Build history of the part. All positions in model axes, mm. Give positions to 0.01 mm unless a question says otherwise; leave off trailing zeros. Order: outer loops, then holes, each group sorted by start corner. A loop starts at its lowest first (then second) coordinate and runs counter-clockwise, first axis right, second up. Notation, with made-up numbers: (-24.5, -28) - (13.5, -28) arc R27 cw to (13.5, -10) - close; hole circle Ø9 at (-27.75, 55). An arc over 180 degrees is marked (long way). Use a Markdown table: item, result. Add a question column.
(1) Slice it at B-B (z = 2.5). Count the separate pieces of the cut face and the enclosed holes in it, then the cut area to 3 significant figures.
(2) Slice it at D-D (x = 23.5). Write the cut outline in (y, z), then the cut area to 3 significant figures.
(3) Wall check: line 1 (X direction, y = 14.25, z = 6.25); line 2 (Y direction, x = 6.5, z = 5.75); line 3 (Y direction, x = 42.5, z = 7). Give the ranges that are in metal, low to high.
(4) Slice it at C-C (y = 23.25). Write the cut outline in (x, z).
(5) Mould opens along Y. For faces 1 (the face through (37.37, 11.62, 3.76)), 2 (the face through (22, 18, 0)), 3 (the face through (22, 28.419, 4)) say: +Y half, -Y half, draft (parallel to the pull), parting line (faces both ways), or undercut.
(6) Slice it at A-A (x = 13.5). Write the cut outline in (y, z), then the cut area to 3 significant figures.
from build123d import *

# Parameters (mm, degrees)
SKETCH1_W           = 45.596558684
SKETCH1_H           = 28.418694735
SKETCH1_R           = 3.675
SKETCH1_R_2         = 3.67
SKETCH1_R_3         = 3.665
SKETCH1_R_4         = 3.66
SKETCH1_R_5         = 3.655
SKETCH1_R_6         = 3.645
SKETCH1_R_7         = 3.64
SKETCH1_R_8         = 3.635
SKETCH1_R_9         = 3.63
SKETCH1_R_10        = 3.62
SKETCH1_R_11        = 3.615
SKETCH1_R_12        = 3.61
SKETCH1_R_13        = 3.605
SKETCH1_R_14        = 3.65
SKETCH1_R_15        = 3.625
BOSS_EXTRUDE1_DEPTH = 7.62
CHAMFER1_SIZE       = 2.54


with BuildPart() as part:
    # Sketch1 → Boss-Extrude1 (new body)
    with BuildSketch(Plane.XY):
        with Locations((22.798279342, 14.209347368)):
            Rectangle(SKETCH1_W, SKETCH1_H)
        with Locations((4.694723918, 4.934387692)):
            Circle(SKETCH1_R, mode=Mode.SUBTRACT)
        with Locations((13.584723918, 4.934387692)):
            Circle(SKETCH1_R_2, mode=Mode.SUBTRACT)
        with Locations((22.474723918, 4.934387692)):
            Circle(SKETCH1_R_3, mode=Mode.SUBTRACT)
        with Locations((31.364723918, 4.934387692)):
            Circle(SKETCH1_R_4, mode=Mode.SUBTRACT)
        with Locations((40.254723918, 4.934387692)):
            Circle(SKETCH1_R_5, mode=Mode.SUBTRACT)
        with Locations((13.584723918, 13.824387692)):
            Circle(SKETCH1_R_6, mode=Mode.SUBTRACT)
        with Locations((22.474723918, 13.824387692)):
            Circle(SKETCH1_R_7, mode=Mode.SUBTRACT)
        with Locations((31.364723918, 13.824387692)):
            Circle(SKETCH1_R_8, mode=Mode.SUBTRACT)
        with Locations((40.254723918, 13.824387692)):
            Circle(SKETCH1_R_9, mode=Mode.SUBTRACT)
        with Locations((13.584723918, 22.714387692)):
            Circle(SKETCH1_R_10, mode=Mode.SUBTRACT)
        with Locations((22.474723918, 22.714387692)):
            Circle(SKETCH1_R_11, mode=Mode.SUBTRACT)
        with Locations((31.364723918, 22.714387692)):
            Circle(SKETCH1_R_12, mode=Mode.SUBTRACT)
        with Locations((40.254723918, 22.714387692)):
            Circle(SKETCH1_R_13, mode=Mode.SUBTRACT)
        with Locations((4.694723918, 13.824387692)):
            Circle(SKETCH1_R_14, mode=Mode.SUBTRACT)
        with Locations((4.694723918, 22.714387692)):
            Circle(SKETCH1_R_15, mode=Mode.SUBTRACT)
    extrude(amount=BOSS_EXTRUDE1_DEPTH)

    # Chamfer1
    chamfer1_edges = [part.edges().sort_by_distance(p)[0] for p in [
        (0, 0, 3.81),
    ]]
    chamfer(chamfer1_edges, length=CHAMFER1_SIZE)


solid = part.part
Solution:
| question | item | result |
|---|---|---|
| 1 | separate pieces | 1 |
| 1 | enclosed holes | 15 |
| 1 | area | 668 mm2 |
| 2 | outline | (0, 0) - (1.42, 0) - (1.42, 7.62) - (0, 7.62) - close; (8.45, 0) - (10.33, 0) - (10.33, 7.62) - (8.45, 7.62) - close; (17.32, 0) - (19.25, 0) - (19.25, 7.62) - (17.32, 7.62) - close; (26.18, 0) - (28.42, 0) - (28.42, 7.62) - (26.18, 7.62) - close |
| 2 | area | 56.9 mm2 |
| 3 | line 1 | 0 to 1.07, 8.32 to 9.96, 17.2 to 18.86, 26.09 to 27.75, 34.97 to 36.65, 43.86 to 45.6 |
| 3 | line 2 | 0 to 1.73, 8.14 to 10.65, 17 to 19.57, 25.86 to 28.42 |
| 3 | line 3 | 0 to 2.05, 7.82 to 10.97, 16.68 to 19.89, 25.53 to 28.42 |
| 4 | outline | (0, 0) - (1.11, 0) - (1.11, 7.62) - (0, 7.62) - close; (8.28, 0) - (10, 0) - (10, 7.62) - (8.28, 7.62) - close; (17.16, 0) - (18.9, 0) - (18.9, 7.62) - (17.16, 7.62) - close; (26.05, 0) - (27.79, 0) - (27.79, 7.62) - (26.05, 7.62) - close; (34.93, 0) - (36.69, 0) - (36.69, 7.62) - (34.93, 7.62) - close; (43.82, 0) - (45.6, 0) - (45.6, 7.62) - (43.82, 7.62) - close |
| 5 | face 1 | undercut |
| 5 | face 2 | draft |
| 5 | face 3 | +Y half |
| 6 | outline | (0, 0) - (1.27, 0) - (1.27, 7.62) - (0, 7.62) - close; (8.6, 0) - (10.18, 0) - (10.18, 7.62) - (8.6, 7.62) - close; (17.47, 0) - (19.1, 0) - (19.1, 7.62) - (17.47, 7.62) - close; (26.33, 0) - (28.42, 0) - (28.42, 7.62) - (26.33, 7.62) - close |
| 6 | area | 49.9 mm2 |
